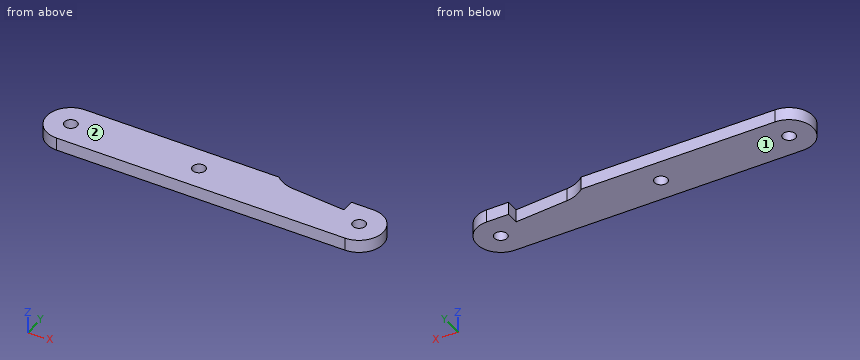
```python
from build123d import *

# Parameters (mm, degrees)
SKETCH1_R           = 2
BOSS_EXTRUDE1_DEPTH = 4
FILLET1_R           = 10


with BuildPart() as part:
    # Sketch1 → Boss-Extrude1 (new body)
    with BuildSketch(Plane.XY):
        with BuildLine():
            Line((0, 7.5), (60.5, 7.5))
            Line((60.5, 7.5), (62.59580051, 5.2))
            Line((62.59580051, 5.2), (83.151712968, 3.5))
            Line((83.151712968, 3.5), (83.151712968, 7.5))
            Line((83.151712968, 7.5), (90, 7.5))
            ThreePointArc((90, 7.5), (97.5, 0), (90, -7.5))
            Line((90, -7.5), (0, -7.5))
            ThreePointArc((0, -7.5), (-7.5, 0), (0, 7.5))
        make_face()
        Circle(SKETCH1_R, mode=Mode.SUBTRACT)
        with Locations((90, 0)):
            Circle(SKETCH1_R, mode=Mode.SUBTRACT)
        with Locations((40, 0)):
            Circle(SKETCH1_R, mode=Mode.SUBTRACT)
    extrude(amount=BOSS_EXTRUDE1_DEPTH)

    # Fillet1
    # the kernel refuses this fillet: 10 mm, written as the material it adds along each edge
    with BuildSketch(Plane(origin=(62.59580051, 5.2, 0), x_dir=(-0.6735330094671406, 0.7391571451038925, 0), z_dir=(0, 0, 1))) as fillet1_piece_1:
        with BuildLine():
            CenterArc((3.972118366, -9.962911125), FILLET1_R, 94.936211763, 37.995780091)
            Line((-2.839179513, -2.641284173), (-2.97540547, -2.494851634))
            Line((-2.97540547, -2.494851634), (-0.136225958, 0.146432539))
            Line((-0.136225958, 0.146432539), (0, 0.2))
            ThreePointArc((0, 0.2), (1.555826129, 0.2), (3.094442936, 0.199258222))
            Line((3.094442936, 0.199258222), (3.111652259, 0))
        make_face()
    extrude(amount=4)


solid = part.part
```
The model under review builds one solid part; all positions refer to its coordinate system, in mm. Face numbers are marked on the shaded views. Round coordinates to 2 decimals unless told otherwise and drop trailing zeros. Loops run counter-clockwise (first coordinate to the right, second up) from the corner with the lowest first, then second, coordinate; pieces in that order, holes last.
Item 1: Take a section at B-B (z = 2.4). Write out the cut boundary in (x, y).
Determined:
outline: (0, -7.5) - (90, -7.5) arc R7.5 ccw to (90, 7.5) - (83.15, 7.5) - (83.15, 3.5) - (66.46, 4.88) arc R10 cw to (60.5, 7.5) - (0, 7.5) arc R7.5 ccw to start; hole circle Ø4 at (0, 0); hole circle Ø4 at (40, 0); hole circle Ø4 at (90, 0)
Item 2: For line 1 (X direction, y = 1.25, z = 2.05); line 2 (X direction, y = 1.75, z = 1.55); line 3 (Y direction, x = 90, z = 1.3), list the stretches that pass through material, from the lowest coordinate up.
Determined:
line 1: x = -7.4 to -1.56, 1.56 to 38.44, 41.56 to 88.44, 91.56 to 97.4
line 2: x = -7.29 to -0.97, 0.97 to 39.03, 40.97 to 89.03, 90.97 to 97.29
line 3: y = -7.5 to -2, 2 to 7.5
Item 3: Mouldability with a two-part tool opening along Z and no side actions: class the marked faces 1 and 2 as released by +Z, released by -Z, zero draft, split by the parting line, or undercut.
Determined:
face 1: released by -Z
face 2: released by +Z
Item 4: Clearance check with flat-ended pins moving along their axes: pin 1 Ø8 at (x, y) = (9.5, 5) entering from -Z; pin 2 Ø1 at (y, z) = (-1, 3) entering from +X; pin 3 Ø2 at (y, z) = (-2.5, 3) entering from -X; pin 4 Ø2 at (y, z) = (5, 2) entering from -X. State where each tip first meets the part, or that it passes through.
Determined:
pin 1: stops at z = 0
pin 2: stops at x = 97.48
pin 3: stops at x = -7.35
pin 4: stops at x = -6.34
Item 5: Take a section at A-A (x = 40). Write out the cut boundary in (y, z), then the cut area to 3 significant figures.
Determined:
outline: (-7.5, 0) - (-2, 0) - (-2, 4) - (-7.5, 4) - close; (2, 0) - (7.5, 0) - (7.5, 4) - (2, 4) - close
area: 44.0 mm2
Item 6: Take a section at C-C (y = 0). Write out the cut boundary in (x, z).
Determined:
outline: (-7.5, 0) - (-2, 0) - (-2, 4) - (-7.5, 4) - close; (2, 0) - (38, 0) - (38, 4) - (2, 4) - close; (42, 0) - (88, 0) - (88, 4) - (42, 4) - close; (92, 0) - (97.5, 0) - (97.5, 4) - (92, 4) - close
